Print and shaded views of the part. All mm, measured from the part's lowest x, y and z. A direction names the side the tool comes from. Give positions to 0.01 mm unless a question says otherwise; leave off trailing zeros. Loops run counter-clockwise (first coordinate to the right, second up) from the corner with the lowest first, then second, coordinate; pieces in that order, holes last. Notation, with made-up numbers: M -20.75,54 L 0.25,54 A7 ccw 0.25,65 Z; hole C 40,-14 d1. An arc over 180 degrees is marked long. Put each result on its own line as item: value. Start each with the question number.
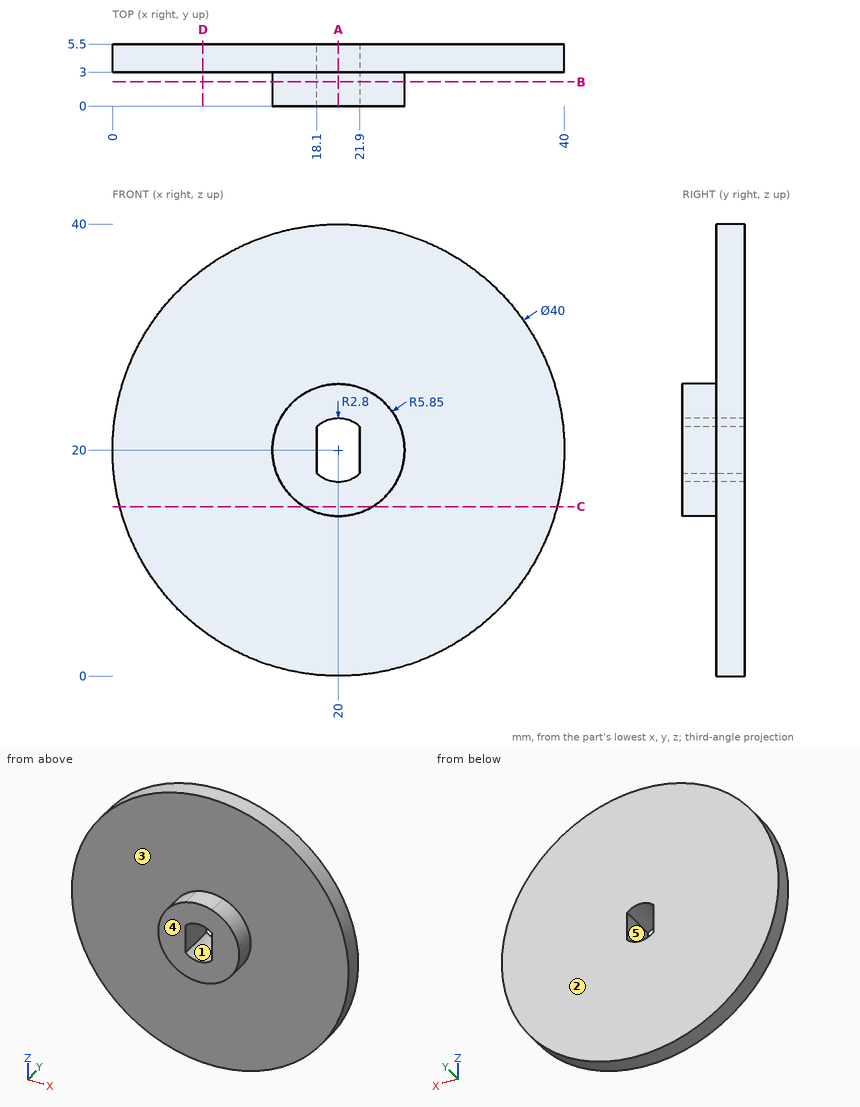
1) Mould opens along Z. For the marked faces 1 and 2 say: +Z half, -Z half, draft (parallel to the pull), parting line (faces both ways), or undercut.
2) Band-saw the part on D-D on x = 8. Give the cut face in (y, z).
3) Wall check: L1, parallel to X at y = 0.7, z = 22.5; L2, parallel to Z at x = 20, y = 2.6; L3, parallel to Y at x = 36, z = 28. Give the ranges that are in metal, low to high.
4) Which spindle directions (+Z, -Z, +X, -X, +Y, -Y) get a long thin tool onto all of the face, cutting with end or side? Do the marked faces 3, 4 and 5. Say none if no direction does.
5) Band-saw the part on A-A on x = 20. Give the cut face in (y, z), then the cut area to 3 significant figures.
6) Band-saw the part on B-B on y = 2.15. Give the cut face in (x, z).
7) Band-saw the part on C-C on z = 15. Give the cut face in (x, y).
8) Pin check, flat tips, straight feed: pin 1 Ø6 at (x, z) = (32, 29.5) entering from -Y; pin 2 Ø1.5 at (y, z) = (4.5, 13.5) entering from -X; pin 3 Ø1.2 at (y, z) = (1.5, 19) entering from +X. Stop position of each tip, or through.
Evaluation:
1. face 1: undercut
1. face 2: draft
2. outline: M 3,4 L 5.5,4 L 5.5,36 L 3,36 Z
3. L1: 14.71 to 18.74, 21.26 to 25.29
3. L2: 14.15 to 17.2, 22.8 to 25.85
3. L3: 3 to 5.5
4. face 3: -Y
4. face 4: +Z, -Z, +X, -X, -Y
4. face 5: +Y, -Y
5. outline: M 0,14.15 L 3,14.15 L 3,0 L 5.5,0 L 5.5,17.2 L 0,17.2 Z; M 0,22.8 L 5.5,22.8 L 5.5,40 L 3,40 L 3,25.85 L 0,25.85 Z
5. area: 104 mm2
6. outline: C 20,20 d11.7; hole M 18.1,17.94 A2.8 ccw 21.9,17.94 L 21.9,22.06 A2.8 ccw 18.1,22.06 Z
7. outline: M 0.64,3 L 16.96,3 L 16.96,0 L 23.04,0 L 23.04,3 L 39.36,3 L 39.36,5.5 L 0.64,5.5 Z
8. pin 1: y = 3
8. pin 2: x = 0.84
8. pin 3: x = 25.84
